Verification items for the finished model (mm, model axes). A direction names the side the tool comes from. Round coordinates to 2 decimals unless told otherwise and drop trailing zeros. Write each loop counter-clockwise with the first axis right and the second up, starting at its lowest first coordinate (ties: lowest second). Pieces come first, ordered by that corner, then holes. Notation, with made-up numbers: (-19, 29) - (28, 29) arc R21 ccw to (28, 54) - close; hole circle Ø7 at (54.25, -28.75). An arc over 180 degrees is marked (long way). Answer as a JSON object with one key per item and string values. Group by question number.
1) Mould release check, pull along Z, two halves, no side actions. Record for faces 6 (the flat face through (25, 5, -17)), 7 (the cylindrical face through (15.54, 8.15, -7.7)), 8 (the flat face through (10, 5, -20)): +Z half, -Z half, draft (parallel to the pull), parting line (faces both ways), or undercut.
2) Set-up check for faces 1 (the flat face through (0, 5, -7)), 2 (the cylindrical face through (2.022, 7.579, -8.984)), 3 (the cylindrical face through (-2.15, 3.44, -17.46)), 4 (the flat face through (10, 6.25, -10)), 5 (the flat face through (20, 5, -7)): record each of +Z, -Z, +X, -X, +Y, -Y from which the full face is reachable in a straight line by a thin tool's end or side.
3) Section check D-D (x = 10). Enter the section's corners in (y, z).
4) Section check B-B (y = 5). Enter the section's corners in (x, z).
5) Section check A-A (x = 22.5). Enter the section's corners in (y, z), then the cut area to 3 significant figures.
6) Thickness scan on line 1 (Y direction, x = -2.5, z = -16.4); line 2 (Z direction, x = 10, y = 7.3); line 3 (X direction, y = 7.75, z = -1.5). Record the ranges inside material, lowest first.
7) Go/stop test with flat-tipped pins: pin 1 Ø3.5 at (x, z) = (8.5, -7) entering from +Y; pin 2 Ø2.5 at (x, y) = (22.5, 6) entering from +Z; pin 3 Ø3 at (y, z) = (6.5, -10) entering from -X; pin 4 Ø3 at (x, y) = (-2.5, 5) entering from +Z. Record where each tip stops, or that it passes through.
8) Section check C-C (y = 1). Enter the section's corners in (x, z), then the cut area to 3 significant figures.
```python
from build123d import *

# Parameters (mm, degrees)
SKETCH1_W           = 20
SKETCH1_H           = 20
BOSS_EXTRUDE1_DEPTH = 10
SKETCH2_R           = 6
CUT_EXTRUDE1_DEPTH  = 3.75
CUT_EXTRUDE3_REACH  = 22
SKETCH5_R           = 1.1
SKETCH6_W           = 5
SKETCH6_H           = 10
BOSS_EXTRUDE2_DEPTH = 5
SKETCH7_R           = 1.6
CUT_EXTRUDE4_DEPTH  = 6


with BuildPart() as part:
    # Sketch1 → Boss-Extrude1 (new body)
    with BuildSketch(Plane(origin=(0, 0, 0), x_dir=(1, 0, 0), z_dir=(0, 1, 0))):
        with Locations((10, 10)):
            Rectangle(SKETCH1_W, SKETCH1_H)
    extrude(amount=BOSS_EXTRUDE1_DEPTH)

    # Sketch2 → Cut-Extrude1 (cut)
    with BuildSketch(Plane(origin=(0, 10, 0), x_dir=(1, 0, 0), z_dir=(0, 1, 0))):
        with Locations((10, 10)):
            Circle(SKETCH2_R)
    extrude(amount=-CUT_EXTRUDE1_DEPTH, mode=Mode.SUBTRACT)

    # Sketch5 → Cut-Extrude3 (cut, up to next)
    with BuildSketch(Plane.ZY, mode=Mode.PRIVATE) as cut_extrude3_sk1:
        with Locations((-10, 8)):
            Circle(SKETCH5_R)
    cut_extrude3_tool1 = extrude(cut_extrude3_sk1.sketch, amount=-CUT_EXTRUDE3_REACH, mode=Mode.PRIVATE) & part.part
    add(cut_extrude3_tool1.solids().sort_by_distance((0, 8, -10))[0], mode=Mode.SUBTRACT)

    # Sketch6 → Boss-Extrude2 (add)
    with BuildSketch(Plane(origin=(20, 0, 0), x_dir=(0, 0, -1), z_dir=(1, 0, 0))):
        with Locations((17.5, 5)):
            Rectangle(SKETCH6_W, SKETCH6_H)
    boss_extrude2 = extrude(amount=BOSS_EXTRUDE2_DEPTH)

    # Sketch7 → Cut-Extrude4 (cut, through all)
    with BuildSketch(Plane.XY.offset(-15)):
        with Locations((22.5, 5)):
            Circle(SKETCH7_R)
    cut_extrude4 = extrude(amount=-CUT_EXTRUDE4_DEPTH, mode=Mode.SUBTRACT)

    # Mirror1: Boss-Extrude2, Cut-Extrude4 across plane
    add(boss_extrude2.mirror(Plane.ZY.offset(-10)))
    add(cut_extrude4.mirror(Plane.ZY.offset(-10)), mode=Mode.SUBTRACT)


solid = part.part
```
Returned:
{
 "1": {"face 6": "draft", "face 7": "undercut", "face 8": "-Z half"},
 "2": {"face 1": "+Z, -X, +Y, -Y", "face 2": "-X", "face 3": "+Z, -Z", "face 4": "+Y", "face 5": "+Z, +X, +Y, -Y"},
 "3": {"outline": "(0, -20) - (10, -20) - (10, -16) - (6.25, -16) - (6.25, -4) - (10, -4) - (10, 0) - (0, 0) - close"},
 "4": {"outline": "(-5, -20) - (-4.1, -20) - (-4.1, -15) - (-5, -15) - close; (-0.9, -20) - (20.9, -20) - (20.9, -15) - (20, -15) - (20, 0) - (0, 0) - (0, -15) - (-0.9, -15) - close; (24.1, -20) - (25, -20) - (25, -15) - (24.1, -15) - close"},
 "5": {"outline": "(0, -20) - (3.4, -20) - (3.4, -15) - (0, -15) - close; (6.6, -20) - (10, -20) - (10, -15) - (6.6, -15) - close", "area": "34.0 mm2"},
 "6": {"line 1": "0 to 3.4, 6.6 to 10", "line 2": "-20 to -16, -4 to 0", "line 3": "0 to 20"},
 "7": {"pin 1": "y = 6.25", "pin 2": "z = -15", "pin 3": "x = 0", "pin 4": "through"},
 "8": {"outline": "(-5, -20) - (25, -20) - (25, -15) - (20, -15) - (20, 0) - (0, 0) - (0, -15) - (-5, -15) - close", "area": "450 mm2"}
}
